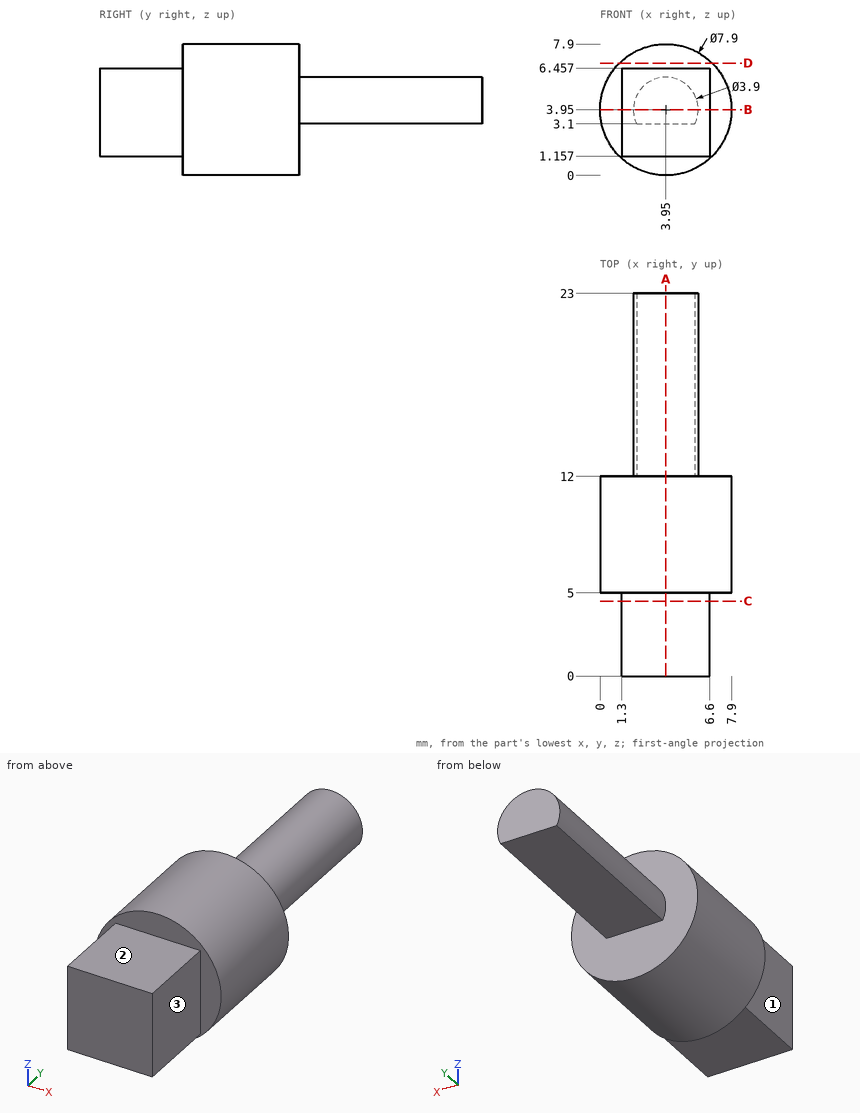
Geometry: see drawing. Coordinates: mm, zero at the bounding-box minimum. A direction names the side the tool comes from. Coordinates: 2 decimals unless noted, no trailing zeros. Write each loop counter-clockwise with the first axis right and the second up, starting at its lowest first coordinate (ties: lowest second). Pieces come first, ordered by that corner, then holes.
1) Section B-B on z = 3.95. Output: boundary loops of the cut face in (x, y), and give its area (3 significant figures).
2) Set-up query: the marked faces 1, 2 and 3. Return all of +Z, -Z, +X, -X, +Y, -Y with unobstructed straight access to the full face (end or side cutting, diameter ignored); none if empty.
3) Section A-A on x = 3.95. Output: boundary loops of the cut face in (y, z), and give its area (3 significant figures).
4) Section D-D on z = 6.75. Output: boundary loops of the cut face in (x, y).
5) Material intervals for line 1 along Y through (x, z) = (7, 2.5); line 2 along X through (y, z) = (1.75, 3.25); line 3 along Z through (x, y) = (2, 1.25), sorted ascending.
6) Pin query (flat end, axial travel): pin 1 Ø1.5 at (x, z) = (2, 1.5) entering from +Y; pin 2 Ø1.5 at (x, y) = (4.5, 1.5) entering from -Z; pin 3 Ø1.5 at (y, z) = (1.5, 2.5) entering from -X. Return the tip coordinate at first contact, or that it passes through.
7) Section C-C on y = 4.5. Output: boundary loops of the cut face in (x, z).
Check result:
1. outline: (0, 5) - (1.3, 5) - (1.3, 0) - (6.6, 0) - (6.6, 5) - (7.9, 5) - (7.9, 12) - (5.9, 12) - (5.9, 23) - (2, 23) - (2, 12) - (0, 12) - close
1. area: 125 mm2
2. face 1: +Z, -Z, -X, -Y
2. face 2: +Z, +X, -X, -Y
2. face 3: +Z, -Z, +X, -Y
3. outline: (0, 1.16) - (5, 1.16) - (5, 0) - (12, 0) - (12, 3.1) - (23, 3.1) - (23, 5.9) - (12, 5.9) - (12, 7.9) - (5, 7.9) - (5, 6.46) - (0, 6.46) - close
3. area: 113 mm2
4. outline: (1.16, 5) - (6.74, 5) - (6.74, 12) - (1.16, 12) - close
5. line 1: y = 5 to 12
5. line 2: x = 1.3 to 6.6
5. line 3: z = 1.16 to 6.46
6. pin 1: stops at y = 12
6. pin 2: stops at z = 1.16
6. pin 3: stops at x = 1.3
7. outline: (1.3, 1.16) - (6.6, 1.16) - (6.6, 6.46) - (1.3, 6.46) - close
